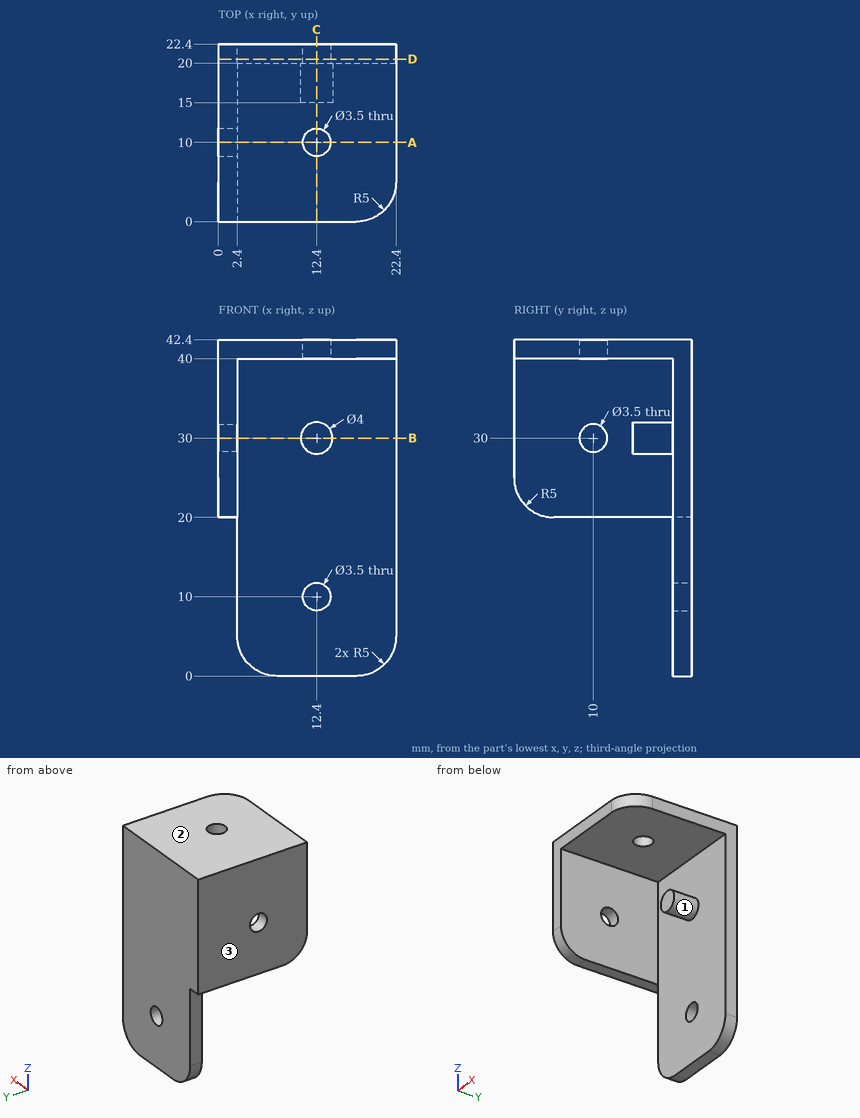
Drawing for the job (mm, zero at the part's lowest x, y, z). Round coordinates to 2 decimals unless told otherwise and drop trailing zeros. Order: outer loops, then holes, each group sorted by start corner. A loop starts at its lowest first (then second) coordinate and runs counter-clockwise, first axis right, second up.
Item 1: Pin check, flat tips, straight feed: pin 1 (1.2 mm diameter, centred on x = 1.5, y = 14, fed in from -Z); pin 2 (1.2 mm diameter, centred on y = 21.5, z = 12, fed in from -X); pin 3 (4.5 mm diameter, centred on x = 11.5, z = 30.5, fed in from -Y); pin 4 (2 mm diameter, centred on x = 12.4, z = 10, fed in from +Y). Stop position of each tip, or through.
Item 2: Saw through at A-A on y = 10. Write the cut outline in (x, z).
Item 3: Saw through at D-D on y = 20.5. Write the cut outline in (x, z).
Item 4: Saw through at C-C on x = 12.4. Write the cut outline in (y, z), then the cut area to 3 significant figures.
Item 5: Mould opens along X. For the marked faces 1, 2 and 3 say: pulls with the +X half, pulls with the -X half, needs draft (parallel to the pull), parting line crosses it, or undercut.
Item 6: Saw through at B-B on z = 30. Write the cut outline in (x, y), then the cut area to 3 significant figures.
Item 7: Probe line 1 along Y through (x, z) = (0.65, 30); line 2 along Z through (x, y) = (12.4, 21.65); line 3 along X through (y, z) = (20.85, 10). List the from-to ranges inside material, lowest first.
Reported:
1. pin 1: stops at z = 20
1. pin 2: stops at x = 2.4
1. pin 3: stops at y = 15
1. pin 4: passes through
2. outline: (0, 20) - (2.4, 20) - (2.4, 28.25) - (0, 28.25) - close; (0, 31.75) - (2.4, 31.75) - (2.4, 40) - (10.65, 40) - (10.65, 42.4) - (0, 42.4) - close; (14.15, 40) - (22.4, 40) - (22.4, 42.4) - (14.15, 42.4) - close
3. outline: (0, 20) - (2.4, 20) - (2.4, 5) arc R5 ccw to (7.4, 0) - (17.4, 0) arc R5 ccw to (22.4, 5) - (22.4, 42.4) - (0, 42.4) - close; hole circle Ø3.5 at (12.4, 10)
4. outline: (0, 40) - (8.25, 40) - (8.25, 42.4) - (0, 42.4) - close; (11.75, 40) - (20, 40) - (20, 32) - (15, 32) - (15, 28) - (20, 28) - (20, 11.75) - (22.4, 11.75) - (22.4, 42.4) - (11.75, 42.4) - close; (20, 0) - (22.4, 0) - (22.4, 8.25) - (20, 8.25) - close
4. area: 153 mm2
5. face 1: undercut
5. face 2: needs draft
5. face 3: pulls with the -X half
6. outline: (0, 0) - (2.4, 0) - (2.4, 8.25) - (0, 8.25) - close; (0, 11.75) - (2.4, 11.75) - (2.4, 20) - (10.4, 20) - (10.4, 15) - (14.4, 15) - (14.4, 20) - (22.4, 20) - (22.4, 22.4) - (0, 22.4) - close
6. area: 113 mm2
7. line 1: y = 0 to 8.25, 11.75 to 22.4
7. line 2: z = 0 to 8.25, 11.75 to 42.4
7. line 3: x = 2.4 to 10.65, 14.15 to 22.4
